CAD build for the part. Positions are in the model's coordinates, mm. Round coordinates to 2 decimals unless told otherwise and drop trailing zeros. Write each loop counter-clockwise with the first axis right and the second up, starting at its lowest first coordinate (ties: lowest second). Pieces come first, ordered by that corner, then holes. Notation, with made-up numbers: (-20, 33.5) -> (37, 33.5) arc R12 ccw to (37, 46.5) -> close; hole circle Ø10 at (56, -2.75). An arc over 180 degrees is marked (long way). Put each result on its own line as item: value. Start each with the question number.
1. Flat gauge pins, fed straight in: P1, Ø1.5, axis at y = 2, z = -16.5, coming from the +X side; P2, Ø2, axis at x = 3.5, y = 3.5, coming from the -Z side. Where does each tip first touch, or does it go through?
2. Drill centre lines: line 1 (Z direction, x = 1.25, y = 2); line 2 (X direction, y = 3.25, z = -7.5); line 3 (Y direction, x = 5, z = -17.25). Where is each one in solid material? Low to high. Write a range as from..to.
3. Pull direction X, two halves, no side cores. Call faces 1 (the flat face through (6.5, 3, 0)), 2 (the flat face through (3, 3, 2.25)), 3 (the cylindrical face through (4.62, 3.13, -2.77)), 4 (the flat face through (0, 3, 0)): pulls with the +X half, pulls with the -X half, needs draft (parallel to the pull), parting line crosses it, or undercut.
4. Saw through at C-C on z = -20. List the corners of the cut face in (x, y), and give its area (3 significant figures).
5. Saw through at A-A on x = 3.5. List the corners of the cut face in (y, z).
Autodesk Inventor part; units mm, degrees
ref_plane "Work Plane1" through (0.2, 3.25, -2.25) normal (0, 1, 0) x (1, 0, 0)
ref_plane "Work Plane2" through (1.5017, 3.2491, -3.5) normal (0, 0, -1) x (-1, 0, 0)
ref_plane "Work Plane3" through (5.0012, 3.2491, -3.5) normal (0, 0, -1) x (-1, 0, 0)
sketch "Sketch1" plane through (0, 0, 0) normal (0, 0, 1) x (1, 0, 0)
  line L0 (0.2, 0) -> (6.3, 0)
  line L1 (6.5, 0.2) -> (6.5, 6.3)
  line L2 (6.3, 6.5) -> (0.2, 6.5)
  line L3 (0, 6.3) -> (0, 0.2)
  arc A0 (0.2, 6.5) -> (0, 6.3) centre (0.2, 6.3) ccw
  arc A1 (6.5, 6.3) -> (6.3, 6.5) centre (6.3, 6.3) ccw
  arc A2 (6.3, 0) -> (6.5, 0.2) centre (6.3, 0.2) ccw
  arc A3 (0, 0.2) -> (0.2, 0) centre (0.2, 0.2) ccw
  point P0 (0, 0)
  point P1 (6.5, 6.5)
  point P2 (6.5, 0)
  point P3 (0, 6.5)
  dimension "d0" = 6.5
  dimension "d1" = 6.5
  dimension "d2" = 0.2
extrude "Extrusion1" add sketch "Sketch1" along normal mid plane 4.5
fillet "Fillet1" radius 0.2 8 edges at (0.0586, 0.0586, 2.25) (3.25, 0, 2.25) (6.4414, 0.0586, 2.25) (6.5, 3.25, 2.25) (6.4414, 6.4414, 2.25) (3.25, 6.5, 2.25) (0.0586, 6.4414, 2.25) (0, 3.25, 2.25)
ref_plane "Work Plane1" through (0.2, 3.25, -2.25) normal (0, 1, 0) x (1, 0, 0)
sketch "Sketch2" plane through (0.2, 3.25, -2.25) normal (0, 1, 0) x (1, 0, 0)
  line L0 (1.3, 0) -> (1.3, 25)
  line L1 (4.8, 0) -> (4.8, 25)
  point P0 (-0.2, -2.25)
  point P1 (-0.2, 0)
  point P2 (6.3, 0)
  dimension "d6" = 1.5
  dimension "d7" = 1.5
  dimension "d8" = 25
  dimension "d9" = 25
sketch "Sketch3" plane through (0, 0, -2.25) normal (0, 0, -1) x (-1, 0, 0)
  circle A0 centre (-1.5017, 3.2491) radius 0.4
  circle A1 centre (-5.0012, 3.2491) radius 0.4
  point P0 (0, 0)
  dimension "d10" = 0.8
  dimension "d11" = 0.8
extrude "Extrusion2" add sketch "Sketch3" along normal blind 1.25 contours A0
extrude "Extrusion3" add sketch "Sketch3" along normal blind 1.25 contours A1
fillet "Fillet2" radius 0.2 2 edges at (1.9017, 3.2491, -3.5) (5.4012, 3.2491, -3.5)
ref_plane "Work Plane2" through (1.5017, 3.2491, -3.5) normal (0, 0, -1) x (-1, 0, 0)
ref_plane "Work Plane3" through (5.0012, 3.2491, -3.5) normal (0, 0, -1) x (-1, 0, 0)
sketch "Sketch4" plane through (1.5017, 3.2491, -3.5) normal (0, 0, -1) x (-1, 0, 0)
  circle A0 centre (0, 0) radius 0.25
  point P0 (1.5017, -3.2491)
  dimension "d19" = 0.5
sketch "Sketch5" plane through (5.0012, 3.2491, -3.5) normal (0, 0, -1) x (-1, 0, 0)
  circle A0 centre (0, 0) radius 0.25
  point P0 (5.0012, -3.2491)
  dimension "d20" = 0.5
sweep "Sweep1" add profiles "Sketch4" path "Sketch2" path curves L0
sweep "Sweep2" add profiles "Sketch5" path "Sketch2" path curves L1
equation "\"BendRadius\" = Thickness"
equation "\"BendReliefWidth\" = Thickness"
equation "\"BendReliefDepth\" = 0.5 * Thickness"
equation "\"CornerReliefSize\" = 4 * Thickness"
equation "\"MinimumRemnant\" = 2 * Thickness"
equation "\"TransitionRadius\" = BendRadius"
equation "\"JacobiRadiusSize\" = BendRadius"
equation "\"GapSize\" = Thickness"
properties part number "KM6A-H90"
Return value:
1. P1: passes through
1. P2: stops at z = -2.25
2. line 1: z = -2.25..2.25
2. line 2: x = 1.25..1.75, 4.75..5.25
2. line 3: y = 3..3.5
3. face 1: pulls with the +X half
3. face 2: needs draft
3. face 3: undercut
3. face 4: pulls with the -X half
4. outline: circle Ø0.5 at (1.5, 3.25); circle Ø0.5 at (5, 3.25)
4. area: 0.393 mm^2
5. outline: (0, -2.25) -> (6.5, -2.25) -> (6.5, 2.05) arc R0.2 ccw to (6.3, 2.25) -> (0.2, 2.25) arc R0.2 ccw to (0, 2.05) -> close
